Autodesk Inventor part; units mm, degrees
ref_plane "YZ Plane" through (0, 0, 0) normal (1, 0, 0) x (0, 1, 0)
ref_plane "XZ Plane" through (0, 0, 0) normal (0, 1, 0) x (-1, 0, 0)
ref_plane "XY Plane" through (0, 0, 0) normal (0, 0, 1) x (1, 0, 0)
sketch "Sketch1" plane through (0, 0, 0) normal (0, 0, 1) x (1, 0, 0)
  line L0 (0, 0) -> (0, 35)
  line L1 (0, 35) -> (3, 35)
  line L2 (3, 28) -> (3, 2)
  line L3 (3, 0) -> (0, 0)
  line L4 (3, 2) -> (6, 2)
  line L5 (6, 2) -> (3, 0)
  line L6 (10, 35) -> (3, 35)
  arc A0 (10, 35) -> (3, 28) centre (11.8151, 26.1849) ccw
  dimension "d7" = 9
  dimension "d8" = 3
  dimension "d9" = 7
  dimension "d10" = 7
extrude "Extrusion1" add sketch "Sketch1" along normal blind 25
fillet "Fillet1" radius 1 1 edges at (0, 17.5, 25)
fillet "Fillet2" radius 1 1 edges at (0, 17.5, 0)
sketch "Sketch2" plane through (3, 0, 0) normal (0, -1, 0) x (1, 0, 0)
  line L0 (-3, 1) -> (-3, 24)
  line L1 (0, 5) -> (-3, 5)
  line L2 (-3, 5) -> (-3, 10)
  line L3 (-3, 10) -> (0, 10)
  line L4 (0, 15) -> (-3, 15)
  line L5 (0, 20) -> (-3, 20)
  line L6 (-3, 15) -> (-3, 20)
  line L7 (3.0852, 20) -> (0, 20)
  line L8 (3.0852, 20) -> (3.0852, 15)
  line L9 (3.0852, 15) -> (-1, 15)
  line L10 (0, 10) -> (1.0426, 10)
  line L11 (1.0426, 10) -> (3.0852, 10)
  line L12 (3.0852, 10) -> (3.0852, 5)
  line L13 (3.0852, 5) -> (0, 5)
  point P0 (-3, 0)
  dimension "d17" = 5
extrude "Extrusion2" cut sketch "Sketch2" against normal blind 5
sketch "Sketch3" plane through (3, 2, 10) normal (0, 1, 0) x (1, 0, 0)
  line L0 (3, 0) -> (0, 0)
  line L1 (0, -5) -> (3, -5)
  line L2 (3, 0) -> (3, -5)
  line L3 (0, -5) -> (0, 0)
  line L4 (3, 0) -> (0, 0)
  line L5 (3, 0) -> (3, -5)
  line L6 (3, -5) -> (0, -5)
  point P0 (-3, 10)
extrude "Extrusion3" cut sketch "Sketch3" against normal blind 5
properties part number "parteA"
Geometry: final body of the model. Coordinates: model frame, mm. A direction names the side the tool comes from. Coordinates: 2 decimals unless noted, no trailing zeros. Order: outer loops, then holes, each group sorted by start corner. A loop starts at its lowest first (then second) coordinate and runs counter-clockwise, first axis right, second up. Notation, with made-up numbers: (35.25, 72) -> (92.25, 72) arc R25 cw to (92.25, 100) -> close; hole circle Ø9 at (32, 45). An arc over 180 degrees is marked (long way). Write item = value, one per line.
(1) Pull-direction query (Z, two-part tool) for faces 1 (the flat face through (2, 2, 5)), 2 (the flat face through (2, 2, 20)), 3 (the flat face through (2, 20, 25)), 4 (the flat face through (4, 2, 2)); classes: pulls with the +Z half, pulls with the -Z half, needs draft (parallel to the pull), parting line crosses it, or undercut.
Solved:
face_1 = undercut
face_2 = undercut
face_3 = pulls with the +Z half
face_4 = needs draft
(2) Line query: line 1 (Z direction, x = 2, y = 4); line 2 (X direction, y = 13, z = 22); line 3 (Y direction, x = 0.5, z = 19.75). Output: solid intervals per line, ascending.
Solved:
line_1 = 0 to 5, 10 to 15, 20 to 25
line_2 = 0 to 3
line_3 = 5 to 35
(3) Pin query (flat end, axial travel): pin 1 Ø5 at (x, y) = (4, 10) entering from +Z; pin 2 Ø3.5 at (x, z) = (2, 8) entering from -Y; pin 3 Ø2 at (y, z) = (26.5, 13) entering from +X. Return the tip coordinate at first contact, or that it passes through.
Solved:
pin_1 = 25
pin_2 = 5
pin_3 = 3
(4) Access query for faces 5 (the flat face through (1, 5, 8)), 6 (the flat face through (4.5, 1, 22.5)), 7 (the flat face through (4, 2, 22)). Directions: +Z, -Z, +X, -X, +Y, -Y. A direction counts if a zero-diameter tool reaches every point of the face in a straight line with its end or side. Return the directions, or none.
Solved:
face_5 = +X, -X, -Y
face_6 = +Z, -Z, +X, -Y
face_7 = +Z, -Z, +X
(5) Cut plane C-C on x = 1.5. Return loops of the section in (y, z), plus the area to 3 significant figures.
Solved:
outline = (0, 0) -> (35, 0) -> (35, 25) -> (0, 25) -> (0, 20) -> (5, 20) -> (5, 15) -> (0, 15) -> (0, 10) -> (5, 10) -> (5, 5) -> (0, 5) -> close
area = 825 mm²
(6) Cut plane A-A on y = 3.5. Return loops of the section in (x, z).
Solved:
outline = (0, 1) arc R1 ccw to (1, 0) -> (3, 0) -> (3, 5) -> (0, 5) -> close; (0, 10) -> (3, 10) -> (3, 15) -> (0, 15) -> close; (0, 20) -> (3, 20) -> (3, 25) -> (1, 25) arc R1 ccw to (0, 24) -> close
(7) Cut plane B-B on z = 20.75. Return loops of the section in (x, y), plus the area to 3 significant figures.
Solved:
outline = (0, 0) -> (3, 0) -> (6, 2) -> (3, 2) -> (3, 28) arc R9 cw to (10, 35) -> (0, 35) -> close
area = 123 mm²
(8) Cut plane D-D on y = 27. Return loops of the section in (x, z).
Solved:
outline = (0, 1) arc R1 ccw to (1, 0) -> (3, 0) -> (3, 25) -> (1, 25) arc R1 ccw to (0, 24) -> close
